from build123d import *

# Parameters (mm, degrees)
F0_R          = 19.05
F1_DEPTH      = 4.7625
F1_DEPTH_BACK = 4.7625
F0_R_2        = 12.7
F2_DEPTH      = 12.7
F2_DEPTH_BACK = 12.7
F3_SIZE       = 1.016
F4_SIZE       = 3.81


with BuildPart() as f1:
    # F0 (on Top) → F1 (new body, two sides)
    with BuildSketch(Plane.XY) as f1_sk:
        with BuildLine():
            Line((-139.7, -28.575), (139.7, -28.575))
            ThreePointArc((139.7, -28.575), (153.170384, -22.995384), (158.75, -9.525))
            Line((158.75, -9.525), (158.75, 9.525))
            ThreePointArc((158.75, 9.525), (153.170384, 22.995384), (139.7, 28.575))
            Line((139.7, 28.575), (-139.7, 28.575))
            ThreePointArc((-139.7, 28.575), (-153.170384, 22.995384), (-158.75, 9.525))
            Line((-158.75, 9.525), (-158.75, -9.525))
            ThreePointArc((-158.75, -9.525), (-153.170384, -22.995384), (-139.7, -28.575))
        make_face()
        with Locations((-133.35, 0)):
            Circle(F0_R, mode=Mode.SUBTRACT)
        with Locations((133.35, 0)):
            Circle(F0_R, mode=Mode.SUBTRACT)
    extrude(amount=F1_DEPTH)
    extrude(f1_sk.sketch, amount=-F1_DEPTH_BACK)

    # F0 (on Top) → F2 (join, two sides)
    with BuildSketch(Plane.XY) as f2_sk:
        with Locations((-133.35, 0)):
            Circle(F0_R)
        with Locations((-133.35, 0)):
            Circle(F0_R_2, mode=Mode.SUBTRACT)
        with Locations((133.35, 0)):
            Circle(F0_R)
        with Locations((133.35, 0)):
            Circle(F0_R_2, mode=Mode.SUBTRACT)
    extrude(amount=F2_DEPTH)
    extrude(f2_sk.sketch, amount=-F2_DEPTH_BACK)

    # F3
    f3_edges = [f1.edges().sort_by_distance(p)[0] for p in [
        (-139.7, -28.575, 0),
        (0, -28.575, 4.7625),
        (139.7, -28.575, 0),
        (0, -28.575, -4.7625),
        (158.75, 0, 4.7625),
        (158.75, 9.525, 0),
        (158.75, 0, -4.7625),
        (158.75, -9.525, 0),
        (0, 28.575, 4.7625),
        (-139.7, 28.575, 0),
        (0, 28.575, -4.7625),
        (139.7, 28.575, 0),
        (-158.75, 9.525, 0),
        (-158.75, 0, 4.7625),
        (-158.75, -9.525, 0),
        (-158.75, 0, -4.7625),
        (120.65, 0, 12.7),
        (146.05, 0, 0),
        (120.65, 0, -12.7),
        (-146.05, 0, 12.7),
        (-120.65, 0, 0),
        (-146.05, 0, -12.7),
        (-152.4, 0, -12.7),
        (114.3, 0, -12.7),
        (114.3, 0, 12.7),
        (-152.4, 0, 12.7),
    ]]
    chamfer(f3_edges, length=F3_SIZE)

    # F4
    f4_edges = [f1.edges().sort_by_distance(p)[0] for p in [
        (-152.4, 0, 4.7625),
        (-152.4, 0, -4.7625),
        (114.3, 0, -4.7625),
        (114.3, 0, 4.7625),
    ]]
    chamfer(f4_edges, length=F4_SIZE)


solid = f1.part
Build history of the part. All positions in model axes, mm. A direction names the side the tool comes from. Round coordinates to 2 decimals unless told otherwise and drop trailing zeros. Write each loop counter-clockwise with the first axis right and the second up, starting at its lowest first coordinate (ties: lowest second). Pieces come first, ordered by that corner, then holes. Notation, with made-up numbers: (52, -39) -> (97, -39) arc R14 cw to (97, -27) -> close; hole circle Ø8 at (-26.75, -12.5). An arc over 180 degrees is marked (long way). Use one line per item in the form item = value.
Q1. Drop flat-ended pins along their axis: P1, Ø23, axis at x = 133.35, y = 0, coming from the -Z side; P2, Ø5, axis at x = 91, y = 11.5, coming from the -Z side; P3, Ø6, axis at x = -35.5, y = 16.5, coming from the +Z side; P4, Ø8, axis at x = 30.5, z = 8, coming from the +Y side. Give the stop position or say it passes through.
Conclusion:
P1 = through
P2 = -4.76
P3 = 4.76
P4 = 28.32
Q2. Band-saw the part on B-B, the plane y = 0. State how many separate pieces and enclosed holes the cut face has, then the cut area to 3 significant figures.
Conclusion:
separate_pieces = 3
enclosed_holes = 0
area = 2,990 mm²
Q3. Two-plate mould, pull along X, no slides. Class faces 1 (the conical face through (151.118, -7.367, 8.388)), 2 (the conical face through (-152.718, -22.259, -4.586)), 3 (the conical face through (151.118, -7.367, -8.388)), 4 (the flat face through (137.3, 13.4, -12.7)): released by +X, released by -X, zero draft, split by the parting line, or undercut.
Conclusion:
face_1 = undercut
face_2 = released by -X
face_3 = undercut
face_4 = zero draft
Q4. Drill centre lines: L1, parallel to X at y = 0.5, z = -8.75; L2, parallel to X at y = 4.5, z = -1; L3, parallel to Y at x = -133.35, z = -8.75. Where is each one in solid material? Low to high.
Conclusion:
L1 = -152.39 to -146.04, -120.66 to -114.31, 114.31 to 120.66, 146.04 to 152.39
L2 = -158.75 to -145.23, -121.47 to 121.47, 145.23 to 158.75
L3 = -19.05 to -12.7, 12.7 to 19.05
Q5. Tool access for faces 5 (the cylindrical face through (114.32, 0.84, -10.11)), 6 (the flat face through (2, 28.575, 0)), 7 (the cylindrical face through (-115.18, 5.72, 10.11)): list every direction of +Z, -Z, +X, -X, +Y, -Y with a clear straight run to the whole face (end or side of a thin tool).
Conclusion:
face_5 = -Z
face_6 = +Z, -Z, +X, -X, +Y
face_7 = +Z
Q6. Band-saw the part on C-C, the plane x = -39. Write the cut outline in (y, z) (1 decimal).
Conclusion:
outline = (-28.6, -3.7) -> (-27.6, -4.8) -> (27.6, -4.8) -> (28.6, -3.7) -> (28.6, 3.7) -> (27.6, 4.8) -> (-27.6, 4.8) -> (-28.6, 3.7) -> close
